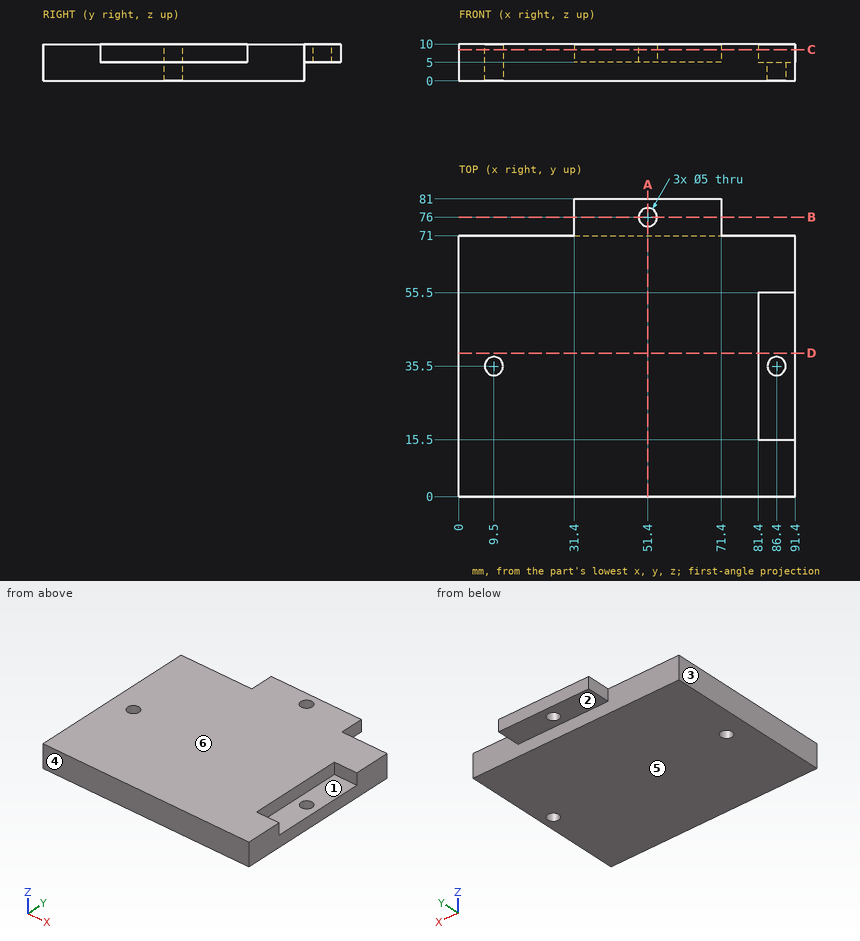
Geometry check sheet. Reference: drawing and pictorial views, mm from the part's lowest x, y, z. A direction names the side the tool comes from. Coordinates: 2 decimals unless noted, no trailing zeros. Order: outer loops, then holes, each group sorted by start corner. A loop starts at its lowest first (then second) coordinate and runs counter-clockwise, first axis right, second up. Notation, with made-up numbers: (12, -25) - (17, -25) arc R11 ccw to (17, -11) - close; hole circle Ø3 at (27, -40). An arc over 180 degrees is marked (long way). Answer in a Markdown table with one row per item. Add a question column.
1) Cross-section at A-A, the plane x = 51.4. Record the cut outline in (y, z), then the cut area to 3 significant figures.
2) Gauge pin test, flat ends, axial feed: P1, Ø8, axis at x = 54, y = 76.5, coming from the -Z side; P2, Ø5, axis at x = 37.5, y = 46.5, coming from the -Z side; P3, Ø8, axis at x = 87, y = 29.5, coming from the +Z side; P4, Ø4, axis at y = 48.5, z = 7.5, coming from the +X side. Record the tip position at first contact, or that the pin passes through.
3) Set-up check for the marked faces 1, 2 and 3: record each of +Z, -Z, +X, -X, +Y, -Y from which the full face is reachable in a straight line by a thin tool's end or side.
4) Material ranges on line 1 along Y through (x, z) = (51.4, 7.15); line 2 along Y through (x, z) = (47.5, 0.5); line 3 along X through (y, z) = (52.5, 8.25), recorded low to high. Write a range as [from, to].
5) Cross-section at B-B, the plane y = 76. Record the cut outline in (x, z).
6) Cross-section at D-D, the plane y = 39. Record the cut outline in (x, z).
7) Release check for a two-part mould opening along Z. For the marked faces 4, 5 and 6 record: +Z half, -Z half, draft (parallel to the pull), parting line (faces both ways), or undercut.
8) Cross-section at C-C, the plane z = 8.5. Record the cut outline in (x, y), then the cut area to 3 significant figures.
Check result:
| question | item | result |
|---|---|---|
| 1 | outline | (0, 0) - (71, 0) - (71, 5) - (73.5, 5) - (73.5, 10) - (0, 10) - close; (78.5, 5) - (81, 5) - (81, 10) - (78.5, 10) - close |
| 1 | area | 735 mm² |
| 2 | P1 | stops at z = 5 |
| 2 | P2 | stops at z = 0 |
| 2 | P3 | stops at z = 5 |
| 2 | P4 | stops at x = 81.4 |
| 3 | face 1 | +Z, +X |
| 3 | face 2 | -Z, +X, -X, +Y |
| 3 | face 3 | +Z, -Z, -X, +Y, -Y |
| 4 | line 1 | y = [0, 73.5], [78.5, 81] |
| 4 | line 2 | y = [0, 71] |
| 4 | line 3 | x = [0, 81.4] |
| 5 | outline | (31.4, 5) - (48.9, 5) - (48.9, 10) - (31.4, 10) - close; (53.9, 5) - (71.4, 5) - (71.4, 10) - (53.9, 10) - close |
| 6 | outline | (0, 0) - (91.4, 0) - (91.4, 5) - (81.4, 5) - (81.4, 10) - (0, 10) - close |
| 7 | face 4 | draft |
| 7 | face 5 | -Z half |
| 7 | face 6 | +Z half |
| 8 | outline | (0, 0) - (91.4, 0) - (91.4, 15.5) - (81.4, 15.5) - (81.4, 55.5) - (91.4, 55.5) - (91.4, 71) - (71.4, 71) - (71.4, 81) - (31.4, 81) - (31.4, 71) - (0, 71) - close; hole circle Ø5 at (9.5, 35.5); hole circle Ø5 at (51.4, 76) |
| 8 | area | 6,450 mm² |
